from build123d import *

# Parameters (mm, degrees)
SKETCH2_R          = 21
SKETCH2_R_2        = 20
CUT_EXTRUDE1_DEPTH = 0.5
FILLET1_R          = 2
CUT_EXTRUDE2_DEPTH = 0.5
CIRPATTERN1_COUNT  = 12


with BuildPart() as part:
    # Sketch1 → Revolve1 (revolve)
    with BuildSketch(Plane(origin=(0, 0, 0), x_dir=(1, 0, 0), z_dir=(0, 1, 0))):
        with BuildLine():
            Line((2, 0), (2, 7.5))
            Line((2, 7.5), (6, 7.5))
            Line((6, 7.5), (6, 3.5))
            Line((6, 3.5), (22, 3.5))
            ThreePointArc((22, 3.5), (23.464737765, 2.015564437), (24, 0))
            Line((24, 0), (2, 0))
        make_face()
    revolve(axis=Axis((0, 0, -79.664313946), (0, 0, 1)))

    # Sketch2 → Cut-Extrude1 (cut)
    with BuildSketch(Plane(origin=(0, 0, -3.5), x_dir=(-1, 0, 0), z_dir=(0, 0, -1))):
        Circle(SKETCH2_R)
        Circle(SKETCH2_R_2, mode=Mode.SUBTRACT)
    extrude(amount=-CUT_EXTRUDE1_DEPTH, mode=Mode.SUBTRACT)

    # Fillet1
    fillet1_edges = [part.edges().sort_by_distance(p)[0] for p in [
        (-22, 0, -3.5),
    ]]
    fillet(fillet1_edges, radius=FILLET1_R)

    # Sketch3 → Cut-Extrude2 (cut)
    with BuildSketch(Plane(origin=(0, 0, -3.5), x_dir=(-1, 0, 0), z_dir=(0, 0, -1))):
        with BuildLine():
            Line((1, 18.723314343), (1, 5.916079783))
            ThreePointArc((1, 5.916079783), (1.552914271, 5.795554958), (2.092014488, 5.623475383))
            Line((2.092014488, 5.623475383), (8.495631768, 16.714865864))
            ThreePointArc((8.495631768, 16.714865864), (4.852857096, 18.111109243), (1, 18.723314343))
        make_face()
    cut_extrude2 = extrude(amount=-CUT_EXTRUDE2_DEPTH, mode=Mode.SUBTRACT)

    # CirPattern1: Cut-Extrude2 ×12 about axis
    cirpattern1_axis = Axis((0, 0, 0), (0, 0, 1))
    for i in range(1, CIRPATTERN1_COUNT):
        add(cut_extrude2.rotate(cirpattern1_axis, i * 360 / CIRPATTERN1_COUNT), mode=Mode.SUBTRACT)

    # Mirror1: part across plane


with BuildPart() as part_1:
    add(part.part)
    add(part.part.mirror(Plane(origin=(2, 0, 0), x_dir=(1, 0, 0), z_dir=(0, 0, -1))))


solid = part_1.part
Part model, mm, in its own coordinate system. A direction names the side the tool comes from. Coordinates: 2 decimals unless noted, no trailing zeros. Order: outer loops, then holes, each group sorted by start corner. A loop starts at its lowest first (then second) coordinate and runs counter-clockwise, first axis right, second up. Notation, with made-up numbers: (-26.75, -38) - (26.25, -38) arc R28 ccw to (26.25, -20) - close; hole circle Ø5 at (81, 24.25). An arc over 180 degrees is marked (long way). Use CSV: the item, a comma, the result in double quotes.
Item 1: Probe probe 1 along Y at (x, z) = (0, 3.3); probe 2 along Y at (x, z) = (0, -3.2); probe 3 along Z at (x, y) = (-10, 9). List the from-to ranges inside material, lowest first.
Solved:
probe 1,"y = -22.22 to -21, -20 to -2, 2 to 20, 21 to 22.22"
probe 2,"y = -22.41 to -21, -20 to -2, 2 to 20, 21 to 22.41"
probe 3,"z = -3 to 3"
Item 2: 3-axis set-ups, long thin cutter, end or side, ignore diameter. For faces 1 (the face through (-4, 14, -3)), 2 (the face through (-14, 4, 3)): which of +Z, -Z, +X, -X, +Y, -Y reach the whole face in a straight line?
Solved:
face 1,"-Z"
face 2,"+Z"
Item 3: Saw through at B-B on z = 2. Give the cut face in (x, y), and give its area (3 significant figures).
Solved:
outline,"circle Ø46.95 at (0, 0); hole circle Ø4 at (0, 0)"
area,"1,720 mm²"
Item 4: Saw through at A-A on z = -4.5. Give the cut face in (x, y), and give its area (3 significant figures).
Solved:
outline,"circle Ø12 at (0, 0); hole circle Ø4 at (0, 0)"
area,"101 mm²"
Item 5: Drop flat-ended pins along their axis: P1, Ø3.5, axis at x = 3, y = -14, coming from the +Z side; P2, Ø0.6, axis at x = -12.5, z = -3.5, coming from the +Y side; P3, Ø3.5, axis at x = 8.5, y = -9.5, coming from the +Z side. Give the stop position or say it passes through.
Solved:
P1,"stops at z = 3"
P2,"stops at y = 18.63"
P3,"stops at z = 3.5"
